The drawing under review shows one solid part. Ordinate dimensions are in mm from its lowest x, y, z. Coordinates: 2 decimals unless noted, no trailing zeros. Loops run counter-clockwise (first coordinate to the right, second up) from the corner with the lowest first, then second, coordinate; pieces in that order, holes last. Notation, with made-up numbers: (-8, -25.75) -> (17, -25.75) arc R11 cw to (17, -5.75) -> close; hole circle Ø10 at (86.5, 63.25). An arc over 180 degrees is marked (long way). Use a Markdown table: item, result.
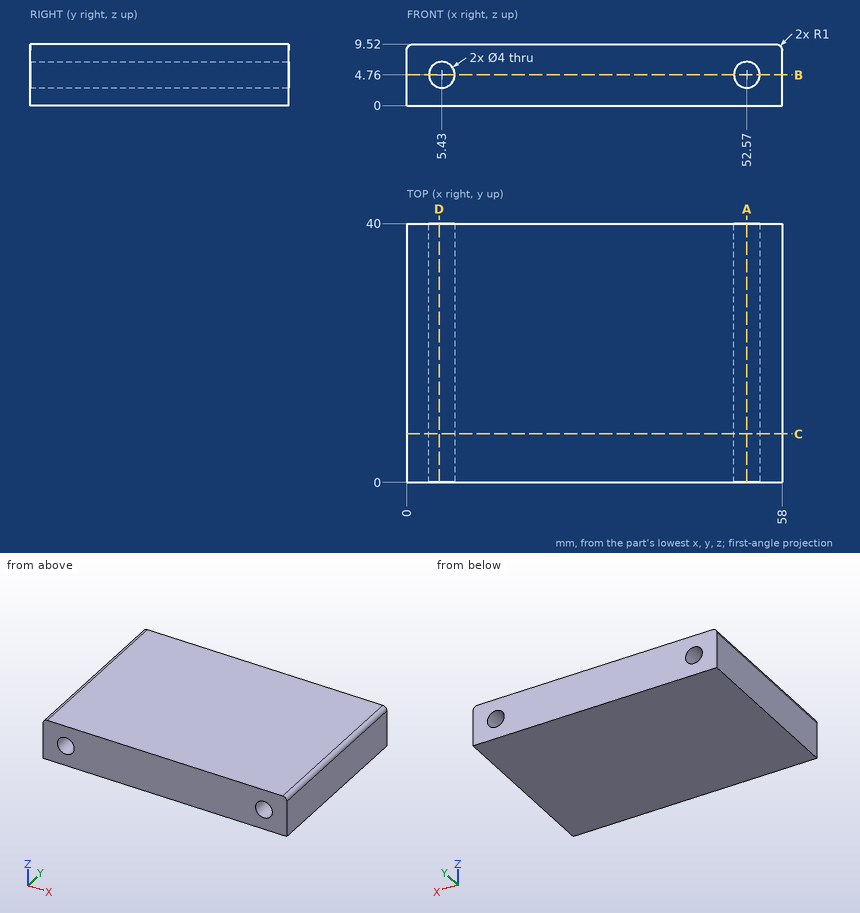
(1) For line 1 along X through (y, z) = (24, 4.75); line 2 along Z through (x, y) = (5.43, 19); line 3 along X through (y, z) = (10, 6), list the stretches that pass through material, from the lowest coordinate up.
Found:
| item | result |
|---|---|
| line 1 | x = 0 to 3.43, 7.43 to 50.57, 54.57 to 58 |
| line 2 | z = 0 to 2.76, 6.76 to 9.52 |
| line 3 | x = 0 to 3.86, 7 to 51, 54.14 to 58 |
(2) Take a section at A-A on x = 52.57. Write out the cut boundary in (y, z), plus the area to 3 significant figures.
Found:
| item | result |
|---|---|
| outline | (0, 0) -> (40, 0) -> (40, 2.76) -> (0, 2.76) -> close; (0, 6.76) -> (40, 6.76) -> (40, 9.52) -> (0, 9.52) -> close |
| area | 221 mm^2 |
(3) For pin 1 Ø1.5 at (y, z) = (20, 7.5) entering from -X, flat-tipped, find the tip position at first contact; note if it passes through.
Found:
| item | result |
|---|---|
| pin 1 | stops at x = 0 |
(4) Take a section at D-D on x = 5. Write out the cut boundary in (y, z), plus the area to 3 significant figures.
Found:
| item | result |
|---|---|
| outline | (0, 0) -> (40, 0) -> (40, 2.81) -> (0, 2.81) -> close; (0, 6.71) -> (40, 6.71) -> (40, 9.52) -> (0, 9.52) -> close |
| area | 225 mm^2 |
(5) Take a section at C-C on y = 7.5. Write out the cut boundary in (x, z), plus the area to 3 significant figures.
Found:
| item | result |
|---|---|
| outline | (0, 0) -> (58, 0) -> (58, 8.52) arc R1 ccw to (57, 9.52) -> (1, 9.52) arc R1 ccw to (0, 8.52) -> close; hole circle Ø4 at (5.43, 4.76); hole circle Ø4 at (52.57, 4.76) |
| area | 527 mm^2 |
(6) Take a section at B-B on z = 4.76. Write out the cut boundary in (x, y), plus the area to 3 significant figures.
Found:
| item | result |
|---|---|
| outline | (0, 0) -> (3.43, 0) -> (3.43, 40) -> (0, 40) -> close; (7.43, 0) -> (50.57, 0) -> (50.57, 40) -> (7.43, 40) -> close; (54.57, 0) -> (58, 0) -> (58, 40) -> (54.57, 40) -> close |
| area | 2,000 mm^2 |
